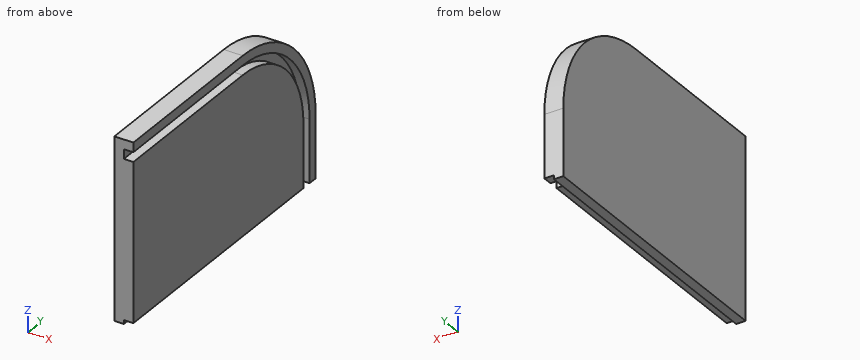
from build123d import *

# Parameters (mm, degrees)
F0_W     = 300
F0_H     = 190
F1_DEPTH = 20
F2_R     = 120
F4_DEPTH = 10
F5_W     = 10
F5_H     = 4
F6_DEPTH = 312


with BuildPart() as f1:
    # F0 (on Right) → F1 (new body)
    with BuildSketch(Plane.YZ):
        with Locations((0.458071, -42.454607)):
            Rectangle(F0_W, F0_H)
    extrude(amount=F1_DEPTH)

    # F2
    f2_edges = [f1.edges().sort_by_distance(p)[0] for p in [
        (10, 150.458071, 52.545393),
    ]]
    fillet(f2_edges, radius=F2_R)

    # F3 (on face) → F4 (cut)
    with BuildSketch(Plane.YZ.offset(20)):
        with BuildLine():
            Line((30.458071, 42.545393), (-149.541929, 42.545393))
            Line((-149.541929, 42.545393), (-149.541929, 32.545393))
            Line((-149.541929, 32.545393), (30.458071, 32.545393))
            ThreePointArc((30.458071, 32.545393), (101.168749, 3.256071), (130.458071, -67.454607))
            Line((130.458071, -67.454607), (130.458071, -137.454607))
            Line((130.458071, -137.454607), (140.458071, -137.454607))
            Line((140.458071, -137.454607), (140.458071, -67.454607))
            ThreePointArc((140.458071, -67.454607), (108.239817, 10.327139), (30.458071, 42.545393))
        make_face()
    extrude(amount=-F4_DEPTH, mode=Mode.SUBTRACT)

    # F5 (on face) → F6 (cut)
    with BuildSketch(Plane.XZ.offset(149.541929)):
        with Locations((15, -135.454607)):
            Rectangle(F5_W, F5_H)
    extrude(amount=-F6_DEPTH, mode=Mode.SUBTRACT)


solid = f1.part
Build history of the part. All positions in model axes, mm. Round coordinates to 2 decimals unless told otherwise and drop trailing zeros. Write each loop counter-clockwise with the first axis right and the second up, starting at its lowest first coordinate (ties: lowest second). Pieces come first, ordered by that corner, then holes. Notation, with made-up numbers: M 15,19 L 24,19 A13 cw 24,36 Z; hole C -39.75,6 d8. An arc over 180 degrees is marked long. Answer in a Markdown table with one row per item.
1. Probe L1, parallel to Z at x = 16.25, y = -96; L2, parallel to Y at x = 10.25, z = -102.5; L3, parallel to Z at x = 12.25, y = 36.5. List the from-to ranges inside material, lowest first. Write a range as [from, to].
Geometry check:
| item | result |
|---|---|
| L1 | [-133.45, 32.55], [42.55, 52.55] |
| L2 | [-149.54, 130.46], [140.46, 150.46] |
| L3 | [-133.45, 32.36], [42.38, 52.39] |
2. Saw through at A-A (x = 16). List the corners of the cut face in (y, z), and give its area (3 significant figures).
Geometry check:
| item | result |
|---|---|
| outline | M -149.54,-133.45 L 130.46,-133.45 L 130.46,-67.45 A100 ccw 30.46,32.55 L -149.54,32.55 Z; M -149.54,42.55 L 30.46,42.55 A110 cw 140.46,-67.45 L 140.46,-133.45 L 150.46,-133.45 L 150.46,-67.45 A120 ccw 30.46,52.55 L -149.54,52.55 Z |
| area | 48,600 mm2 |
3. Flat gauge pins, fed straight in: P1, Ø3, axis at x = 17.5, y = -12.5, coming from the -Z side; P2, Ø5, axis at x = 17, y = 73.5, coming from the +Z side; P3, Ø1, axis at x = 14.5, z = -15, coming from the +Y side. Where does each tip first touch, or does it go through?
Geometry check:
| item | result |
|---|---|
| P1 | z = -133.45 |
| P2 | z = 45.49 |
| P3 | y = 138.63 |
4. Saw through at C-C (y = -74). List the corners of the cut face in (x, z), and give its area (3 significant figures).
Geometry check:
| item | result |
|---|---|
| outline | M 0,-137.45 L 10,-137.45 L 10,-133.45 L 20,-133.45 L 20,32.55 L 10,32.55 L 10,42.55 L 20,42.55 L 20,52.55 L 0,52.55 Z |
| area | 3,660 mm2 |
5. Saw through at B-B (z = -105). List the corners of the cut face in (x, y), and give its area (3 significant figures).
Geometry check:
| item | result |
|---|---|
| outline | M 0,-149.54 L 20,-149.54 L 20,130.46 L 10,130.46 L 10,140.46 L 20,140.46 L 20,150.46 L 0,150.46 Z |
| area | 5,900 mm2 |
6. Saw through at D-D (z = -13). List the corners of the cut face in (x, y).
Geometry check:
| item | result |
|---|---|
| outline | M 0,-149.54 L 20,-149.54 L 20,114.33 L 10,114.33 L 10,126.03 L 20,126.03 L 20,137.39 L 0,137.39 Z |
